from build123d import *

# Parameters (mm, degrees)
BOSS_EXTRUDE1_DEPTH = 125
SKETCH2_R           = 1.9
CUT_EXTRUDE1_DEPTH  = 131.893086143
SKETCH3_W           = 8
SKETCH3_H           = 4
CUT_EXTRUDE2_DEPTH  = 130.761319352


with BuildPart() as part:
    # Sketch1 → Boss-Extrude1 (new body)
    with BuildSketch(Plane.XY):
        Polygon((11, 5), (-11, 5), (-11, -5), (-16, -5), (-16, -22), (-6, -22), (-6, -17), (-11, -17), (-11, -10), (11, -10), (11, -17), (6, -17), (6, -22), (16, -22), (16, -5), (11, -5), align=None)
    extrude(amount=-BOSS_EXTRUDE1_DEPTH)

    # Sketch2 → Cut-Extrude1 (cut, through all)
    with BuildSketch(Plane(origin=(16, 0, 0), x_dir=(0, 0, -1), z_dir=(1, 0, 0))):
        with Locations((62.5, -13.5)):
            Circle(SKETCH2_R)
        with Locations((79.5, -13.5)):
            Circle(SKETCH2_R)
        with Locations((96.5, -13.5)):
            Circle(SKETCH2_R)
        with Locations((45.5, -13.5)):
            Circle(SKETCH2_R)
        with Locations((28.5, -13.5)):
            Circle(SKETCH2_R)
        with Locations((113.5, -13.5)):
            Circle(SKETCH2_R)
        with Locations((11.5, -13.5)):
            Circle(SKETCH2_R)
    extrude(amount=-CUT_EXTRUDE1_DEPTH, mode=Mode.SUBTRACT)

    # Sketch3 → Cut-Extrude2 (cut, through all)
    with BuildSketch(Plane(origin=(11, 0, 0), x_dir=(0, 0, -1), z_dir=(1, 0, 0))):
        with Locations((79.5, 0)):
            Rectangle(SKETCH3_W, SKETCH3_H)
        with Locations((62.5, 0)):
            Rectangle(SKETCH3_W, SKETCH3_H)
        with Locations((96.5, 0)):
            Rectangle(SKETCH3_W, SKETCH3_H)
        with Locations((45.5, 0)):
            Rectangle(SKETCH3_W, SKETCH3_H)
        with Locations((28.5, 0)):
            Rectangle(SKETCH3_W, SKETCH3_H)
        with Locations((113.5, 0)):
            Rectangle(SKETCH3_W, SKETCH3_H)
        with Locations((11.5, 0)):
            Rectangle(SKETCH3_W, SKETCH3_H)
    extrude(amount=-CUT_EXTRUDE2_DEPTH, mode=Mode.SUBTRACT)


solid = part.part
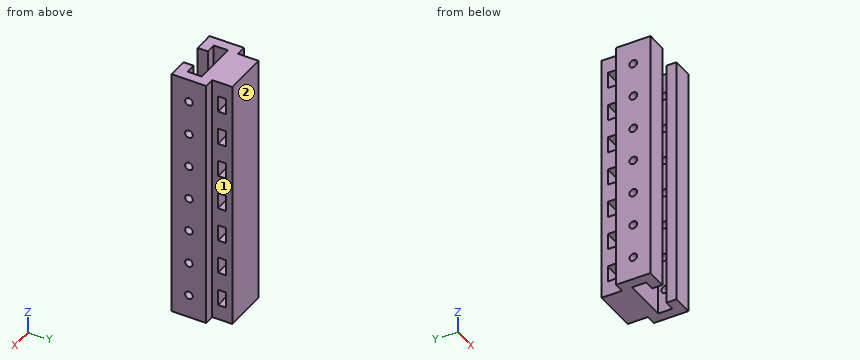
CAD build for the part. Positions are in the model's coordinates, mm. Face numbers are marked on the shaded views. A direction names the side the tool comes from. Round coordinates to 2 decimals unless told otherwise and drop trailing zeros. Order: outer loops, then holes, each group sorted by start corner. A loop starts at its lowest first (then second) coordinate and runs counter-clockwise, first axis right, second up. Notation, with made-up numbers: (53.25, -19) -> (111.25, -19) arc R30 ccw to (111.25, 14) -> close; hole circle Ø10 at (15.5, 30). An arc over 180 degrees is marked (long way). Write item = value, one per line. Start each with the question number.
(1) Pin check, flat tips, straight feed: P1, Ø5, axis at y = 0, z = -55.5, coming from the +X side; P2, Ø6.5, axis at x = -2.5, z = -81.5, coming from the -Y side; P3, Ø3, axis at y = -13.5, z = -28.5, coming from the +X side; P4, Ø3, axis at x = -4, y = 0, coming from the +Z side. Stop position of each tip, or through.
(2) Cut at B-B, the plane x = -8. State how many separate pieces and enclosed holes the cut face has, then the cut area to 3 significant figures.
(3) Cut at D-D, the plane z = -90. List the corners of the cut face in (x, y).
(4) Cut at A-A, the plane z = -28.5. List the corners of the cut face in (x, y).
(5) Probe line 1 (Y direction, x = -7.5, z = -112); line 2 (Y direction, x = -7.5, z = -19.5); line 3 (Y direction, x = 13.6, z = -11.5). List the from-to ranges inside material, lowest first. Write a range as [from, to].
(6) Which spindle directions (+Z, -Z, +X, -X, +Y, -Y) get a long thin tool onto all of the face, cutting with end or side? Do the marked faces 1 and 2. Say none if no direction does.
Model answer:
q1.P1 = 11
q1.P2 = -10
q1.P3 = through
q1.P4 = 0
q2.separate_pieces = 2
q2.enclosed_holes = 7
q2.area = 2,280 mm2
q3.outline = (-16, -22) -> (-6, -22) -> (-6, -17) -> (-11, -17) -> (-11, -10) -> (11, -10) -> (11, -17) -> (6, -17) -> (6, -22) -> (16, -22) -> (16, -5) -> (11, -5) -> (11, 5) -> (-11, 5) -> (-11, -5) -> (-16, -5) -> close
q4.outline = (-16, -22) -> (-6, -22) -> (-6, -17) -> (-11, -17) -> (-11, -15.4) -> (-16, -15.4) -> close; (-16, -11.6) -> (-11, -11.6) -> (-11, -10) -> (11, -10) -> (11, -11.6) -> (16, -11.6) -> (16, -5) -> (11, -5) -> (11, -2) -> (-11, -2) -> (-11, -5) -> (-16, -5) -> close; (-11, 2) -> (11, 2) -> (11, 5) -> (-11, 5) -> close; (6, -22) -> (16, -22) -> (16, -15.4) -> (11, -15.4) -> (11, -17) -> (6, -17) -> close
q5.line_1 = [-22, -17], [-10, -2], [2, 5]
q5.line_2 = [-22, -17], [-10, 5]
q5.line_3 = [-22, -15.4], [-11.6, -5]
q6.face_1 = +Z, -Z, +X, +Y
q6.face_2 = +Z, -Z, +X, -X, +Y
